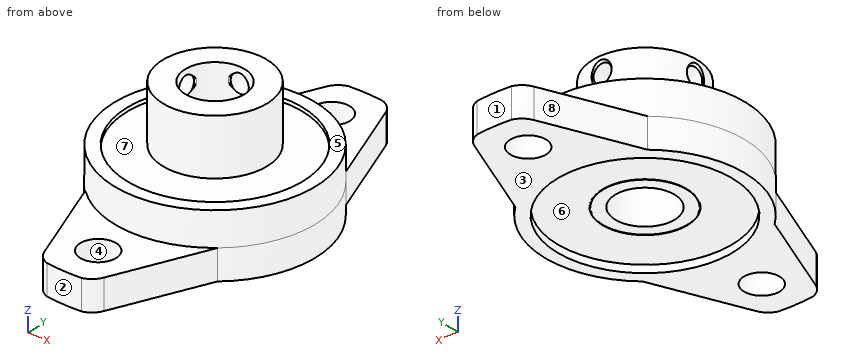
Autodesk Inventor part; units mm, degrees
ref_plane "to_screw_XY" through (0, 4, 6) normal (0, 1, 0) x (1, 0, 0)
ref_plane "to_screw_YZ" through (0, 4, 6) normal (1, 0, 0) x (0, 0, -1)
ref_plane "to_screw_ZX" through (0, 4, 6) normal (0, 0, -1) x (0, 1, 0)
sketch "Sketch_1" plane through (0, 0, 0) normal (1, 0, 0) x (0, 1, 0)
  line L0 (0, -8) -> (0, 8)
  line L1 (7, 8) -> (4, 8)
  line L2 (4, 8) -> (4, -7)
  line L3 (4, -7) -> (5.6375, -7)
  arc A0 (5.7375, -7) -> (5.6375, -7) centre (5.6875, -7) ccw
  line L4 (5.7375, -7) -> (11.8125, -7)
  line L5 (11.8125, -7) -> (11.8125, -8)
  line L6 (11.8125, -8) -> (24, -8)
  line L7 (24, -8) -> (24, -4)
  line L8 (24, -4) -> (13.5, -4)
  line L9 (13.5, -4) -> (13.5, 0.5)
  line L10 (13.5, 0.5) -> (11.8125, 0.5)
  line L11 (11.8125, 0.5) -> (11.8125, 0)
  line L12 (11.8125, 0) -> (5.6875, 0)
  line L13 (5.6875, 0) -> (5.6875, 0.5)
  line L14 (5.6875, 0.5) -> (7, 0.5)
  line L15 (7, 0.5) -> (7, 8)
revolve "Revolution1" add sketch "Sketch_1" angle 360 about axis through (0, 0, -8) along (0, 0, -1)
sketch "Sketch_2" plane through (0, 0, 0) normal (0, 0, 1) x (1, 0, 0)
  line L0 (-54, -96) -> (54, -96)
  line L1 (54, -96) -> (54, 96)
  line L2 (54, 96) -> (-54, 96)
  line L3 (-54, 96) -> (-54, -96)
  arc A0 (-9, 10.0623) -> (-9, -10.0623) centre (0, 0) ccw
  line L4 (-9, -10.0623) -> (-4.0569, -22.3105)
  arc A1 (-4.0569, -22.3105) -> (-1.5531, -24) centre (-1.5531, -21.3) ccw
  line L5 (-1.5531, -24) -> (1.5531, -24)
  arc A2 (1.5531, -24) -> (4.0569, -22.3105) centre (1.5531, -21.3) ccw
  line L6 (4.0569, -22.3105) -> (9, -10.0623)
  arc A3 (9, -10.0623) -> (9, 10.0623) centre (0, 0) ccw
  line L7 (9, 10.0623) -> (4.0569, 22.3105)
  arc A4 (4.0569, 22.3105) -> (1.5531, 24) centre (1.5531, 21.3) ccw
  line L8 (1.5531, 24) -> (-1.5531, 24)
  arc A5 (-1.5531, 24) -> (-4.0569, 22.3105) centre (-1.5531, 21.3) ccw
  line L9 (-4.0569, 22.3105) -> (-9, 10.0623)
extrude "Extrusion1" cut sketch "Sketch_2" along normal mid plane 32
sketch "Sketch_3" plane through (0, 0, 0) normal (1, 0, 0) x (0, 1, 0)
  line L0 (18.5, -8) -> (18.5, 8)
  line L1 (18.5, 8) -> (22.34, 8)
  line L2 (22.34, 8) -> (22.34, -4)
  line L3 (22.34, -4) -> (20.9, -4)
  line L4 (20.9, -4) -> (20.9, -8)
  line L5 (20.9, -8) -> (18.5, -8)
  line L6 (18.5, -8) -> (18.5, 8)
revolve "Revolution2" cut sketch "Sketch_3" angle 360 about axis through (0, 18.5, -8) along (0, 0, -1)
sketch "Sketch_4" plane through (0, 0, 0) normal (1, 0, 0) x (0, 1, 0)
  line L0 (-18.5, -8) -> (-18.5, 8)
  line L1 (-18.5, 8) -> (-14.66, 8)
  line L2 (-14.66, 8) -> (-14.66, -4)
  line L3 (-14.66, -4) -> (-16.1, -4)
  line L4 (-16.1, -4) -> (-16.1, -8)
  line L5 (-16.1, -8) -> (-18.5, -8)
  line L6 (-18.5, -8) -> (-18.5, 8)
revolve "Revolution3" cut sketch "Sketch_4" angle 360 about axis through (0, -18.5, -8) along (0, 0, -1)
sketch "Sketch_5" plane through (0, 0, 0) normal (1, 0, 0) x (0, 1, 0)
  line L0 (3.65, 6) -> (7, 6)
  line L1 (7, 6) -> (7, 4.5)
  line L2 (7, 4.5) -> (6.7295, 4.7705)
  line L3 (6.7295, 4.7705) -> (3.9205, 4.7705)
  line L4 (3.9205, 4.7705) -> (3.65, 4.5)
  line L5 (3.65, 4.5) -> (3.65, 6)
  line L6 (3.65, 6) -> (7, 6)
revolve "Revolution4" cut sketch "Sketch_5" angle 360 about axis through (0, 3.65, 6) along (0, -1, 0)
thread "Thread1"
sketch "Sketch_6" plane through (0, 0, 0) normal (0, 1, 0) x (-1, 0, 0)
  line L0 (7, 6) -> (3.65, 6)
  line L1 (3.65, 6) -> (3.65, 7.5)
  line L2 (3.65, 7.5) -> (3.9205, 7.2295)
  line L3 (3.9205, 7.2295) -> (6.7295, 7.2295)
  line L4 (6.7295, 7.2295) -> (7, 7.5)
  line L5 (7, 7.5) -> (7, 6)
  line L6 (7, 6) -> (3.65, 6)
revolve "Revolution5" cut sketch "Sketch_6" angle 360 about axis through (-7, 0, 6) along (-1, 0, 0)
thread "Thread2"
ref_plane "to_screw_XY" through (0, 4, 6) normal (0, 1, 0) x (1, 0, 0)
ref_plane "to_screw_YZ" through (0, 4, 6) normal (1, 0, 0) x (0, 0, -1)
ref_plane "to_screw_ZX" through (0, 4, 6) normal (0, 0, -1) x (0, 1, 0)
ref_plane "to_screw_2_XY" through (-4, 0, 6) normal (-1, 0, 0) x (0, 0, -1)
ref_plane "to_screw_2_YZ" through (-4, 0, 6) normal (0, 0, -1) x (0, -1, 0)
ref_plane "to_screw_2_ZX" through (-4, 0, 6) normal (0, -1, 0) x (-1, 0, 0)
properties part number "HBR8x"
Input: part model. Units: mm. Frame: model coordinates. Face numbers are marked on the shaded views. A direction names the side the tool comes from. Give positions to 0.01 mm unless a question says otherwise; leave off trailing zeros. Order: outer loops, then holes, each group sorted by start corner. A loop starts at its lowest first (then second) coordinate and runs counter-clockwise, first axis right, second up. Notation, with made-up numbers: (83.5, -14) - (88.5, -14) arc R23 ccw to (88.5, 18) - close; hole circle Ø7 at (63, -8). An arc over 180 degrees is marked (long way). Put each result on its own line as item: value.
Item 1: Section query A-A, the plane z = 6. Return loops of the section in (x, y).
Found:
outline: (-6.87, -1.37) arc R7 ccw (long way) to (1.37, 6.87) - (1.23, 6.73) - (1.23, 3.92) - (1.4, 3.75) arc R4 cw (long way) to (-3.75, -1.4) - (-3.92, -1.23) - (-6.73, -1.23) - close; (-6.87, 1.37) - (-6.73, 1.23) - (-3.92, 1.23) - (-3.75, 1.4) arc R4 cw to (-1.4, 3.75) - (-1.23, 3.92) - (-1.23, 6.73) - (-1.37, 6.87) arc R7 ccw to start
Item 2: Section query C-C, the plane x = -8. Return loops of the section in (y, z), then the cut area to 3 significant figures.
Found:
outline: (-12.54, -8) - (-8.69, -8) - (-8.69, -7) - (8.69, -7) - (8.69, -8) - (12.54, -8) - (12.54, -4) - (10.87, -4) - (10.87, 0.5) - (8.69, 0.5) - (8.69, 0) - (-8.69, 0) - (-8.69, 0.5) - (-10.87, 0.5) - (-10.87, -4) - (-12.54, -4) - close
area: 172 mm^2
Item 3: Section query D-D, the plane y = 8. Return loops of the section in (x, z), then the cut area to 3 significant figures.
Found:
outline: (-10.87, -8) - (-8.69, -8) - (-8.69, -7) - (8.69, -7) - (8.69, -8) - (10.87, -8) - (10.87, 0.5) - (8.69, 0.5) - (8.69, 0) - (-8.69, 0) - (-8.69, 0.5) - (-10.87, 0.5) - close
area: 159 mm^2
Item 4: Ray query, L1, parallel to Z at x = 0, y = 5.9; L2, parallel to X at y = 0, z = 4.5; L3, parallel to X at y = 0, z = -1.75. Return the intervals inside material, ascending. Write a range as from..to.
Found:
L1: z = -7..0, 0.5..4.77, 7.23..8
L2: x = -7..-4, 4..7
L3: x = -13.5..-4, 4..13.5
Item 5: Section query B-B, the plane y = 18.5. Return loops of the section in (x, z).
Found:
outline: (-5.59, -8) - (-2.4, -8) - (-2.4, -4) - (-5.59, -4) - close; (2.4, -8) - (5.59, -8) - (5.59, -4) - (2.4, -4) - close
Item 6: Contact query for flat-ended pins moving along their axis: pin 1 (5 mm diameter, centred on x = -3, z = 0.5, fed in from -Y); pin 2 (4 mm diameter, centred on x = 0, y = -18.5, fed in from -Z); pin 3 (2 mm diameter, centred on x = -7.5, z = 1, fed in from -Y); pin 4 (10 mm diameter, centred on x = -3, y = 2, fed in from -Z). Output: stop coordinate, or through.
Found:
pin 1: stops at y = -13.49
pin 2: passes through
pin 3: stops at y = -11.76
pin 4: stops at z = -7
Item 7: Access query for the marked faces 5, 6, 7 and 8. Directions: +Z, -Z, +X, -X, +Y, -Y. A direction counts if a zero-diameter tool reaches every point of the face in a straight line with its end or side. Return the directions, or none.
Found:
face 5: +Z
face 6: -Z
face 7: none
face 8: +Z, -Z, -X, +Y
Item 8: Draft query along Y for the marked faces 1, 2, 3 and 4. Return one class per face: +Y half, -Y half, draft (parallel to the pull), parting line (faces both ways), or undercut.
Found:
face 1: +Y half
face 2: -Y half
face 3: draft
face 4: undercut
